```python
from build123d import *

# Parameters (mm, degrees)
SKETCH1_R           = 2.6289
BOSS_EXTRUDE1_DEPTH = 6.35
SKETCH2_R           = 4.7625
CUT_EXTRUDE1_DEPTH  = 6.35


with BuildPart() as part:
    # Sketch1 → Boss-Extrude1 (new body)
    with BuildSketch(Plane.XY):
        with BuildLine():
            Line((177.8, -57.15), (228.6, -57.15))
            ThreePointArc((228.6, -57.15), (205.049978384, -116.097324969), (166.619450395, -166.619450395))
            Line((166.619450395, -166.619450395), (132.058628079, -132.058628079))
            ThreePointArc((132.058628079, -132.058628079), (159.392339806, -97.32956648), (177.8, -57.15))
        make_face()
        with Locations((190.5, -69.85)):
            Circle(SKETCH1_R, mode=Mode.SUBTRACT)
        with Locations((215.9, -69.85)):
            Circle(SKETCH1_R, mode=Mode.SUBTRACT)
        with Locations((158.319295358, -140.358783116)):
            Circle(SKETCH1_R, mode=Mode.SUBTRACT)
    extrude(amount=BOSS_EXTRUDE1_DEPTH)

    # Sketch2 → Cut-Extrude1 (cut)
    with BuildSketch(Plane.XY.offset(6.35)):
        with Locations((193.77605394, -134.07059118)):
            Circle(SKETCH2_R)
        with Locations((214.661540739, -97.182845336)):
            Circle(SKETCH2_R)
    extrude(amount=-CUT_EXTRUDE1_DEPTH, mode=Mode.SUBTRACT)


solid = part.part
```
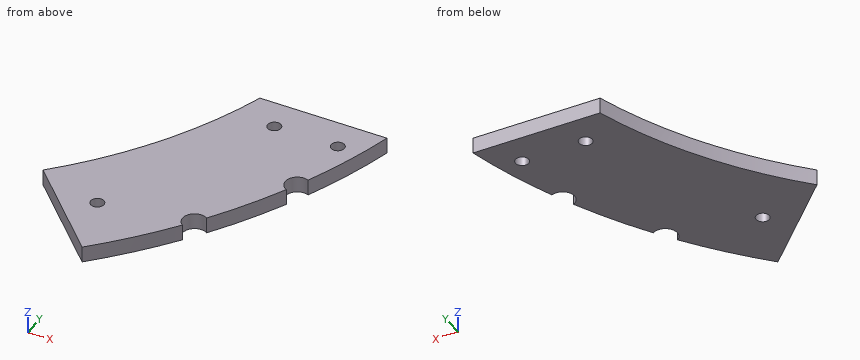
Input: part model. Units: mm. Frame: model coordinates. Round coordinates to 2 decimals unless told otherwise and drop trailing zeros. Write each loop counter-clockwise with the first axis right and the second up, starting at its lowest first coordinate (ties: lowest second). Pieces come first, ordered by that corner, then holes. Notation, with made-up numbers: M -18,51.25 L 31,51.25 A13 ccw 31,66.25 Z; hole C -4.5,61 d6. An arc over 180 degrees is marked long. Write each question's results on one line, items separated by ' | '.
Q1. Section query A-A (y = -69.85). Return loops of the section in (x, z), and give its area (3 significant figures).
Results:
outline: M 173.2,0 L 187.87,0 L 187.87,6.35 L 173.2,6.35 Z; M 193.13,0 L 213.27,0 L 213.27,6.35 L 193.13,6.35 Z; M 218.53,0 L 225.04,0 L 225.04,6.35 L 218.53,6.35 Z | area: 262 mm^2
Q2. Section query C-C (x = 173). Return loops of the section in (y, z), and give its area (3 significant figures).
Results:
outline: M -159.98,0 L -70.36,0 L -70.36,6.35 L -159.98,6.35 Z | area: 569 mm^2
Q3. Line query: line 1 along Y through (x, z) = (190.5, 5); line 2 along Y through (x, z) = (215.5, 3.5); line 3 along Y through (x, z) = (215.9, 2.5). Output: solid intervals per line, ascending.
Results:
line 1: y = -138.69 to -137.53, -130.61 to -72.48, -67.22 to -57.15 | line 2: y = -92.49 to -72.45, -67.25 to -57.15 | line 3: y = -92.58 to -72.48, -67.22 to -57.15
Q4. Pin query (flat end, axial travel): P1, Ø6, axis at x = 158.32, y = -140.36, coming from the -Z side; P2, Ø1, axis at x = 203, z = 5.5, coming from the -Y side; P3, Ø1.5, axis at y = -76, z = 5.5, coming from the -X side; P4, Ø3, axis at x = 151, z = 4.5, coming from the +Y side. Return the tip coordinate at first contact, or that it passes through.
Results:
P1: stops at z = 0 | P2: stops at y = -120.49 | P3: stops at x = 170.26 | P4: stops at y = -107.81
Q5. Section query B-B (z = 1.5). State how many separate pieces and enclosed holes the cut face has, and give its area (3 significant figures).
Results:
separate pieces: 1 | enclosed holes: 3 | area: 5,140 mm^2
Q6. Section query D-D (y = -81). Return loops of the section in (x, z), and give its area (3 significant figures).
Results:
outline: M 168.28,0 L 221.28,0 L 221.28,6.35 L 168.28,6.35 Z | area: 337 mm^2
